The figure shows three views and two pictorial views of one solid part (mm, origin at its lowest corner). Answer the questions. A direction names the side the tool comes from. Coordinates: 2 decimals unless noted, no trailing zeros. Loops run counter-clockwise (first coordinate to the right, second up) from the corner with the lowest first, then second, coordinate; pieces in that order, holes last. Notation, with made-up numbers: (-3.5, 62) - (26.5, 62) arc R22 cw to (26.5, 101) - close; hole circle Ø2 at (28, 42). An arc over 180 degrees is marked (long way). Return JSON: item names as keys, results as strings. Group by question number.
1. Section A-A (z = 18) is taken. Write down the section's boundary in (x, y).
2. Each of these flat-tipped pins is pushed along its axis until it touches: P1, Ø2, axis at x = 8, z = 22, coming from the +Y side; P2, Ø10, axis at x = 27, y = 10, coming from the +Z side; P3, Ø4, axis at x = 27.5, y = 18, coming from the +Z side. Where does it stop, or does it pass through?
3. The mould has two halves that part along Y. Classify the marked faces 1, 2, 3 and 4: pulls with the +Y half, pulls with the -Y half, needs draft (parallel to the pull), parting line crosses it, or undercut.
4. Section C-C (x = 16) is taken. Write down the section's boundary in (y, z).
5. Section D-D (z = 3) is taken. Write down the section's boundary in (x, y).
6. Find the intervals of material crossed by line 1 along Y through (x, z) = (15, 3); line 2 along X through (y, z) = (7.5, 31); line 3 along X through (y, z) = (3, 19.5), in increasing order.
7. Which of the six approach directions +Z, -Z, +X, -X, +Y, -Y give full straight-line access (tool end or side, diameter ignored) to the marked faces 5, 6 and 7?
8. Section B-B (y = 17.5) is taken. Write down the section's boundary in (x, z).
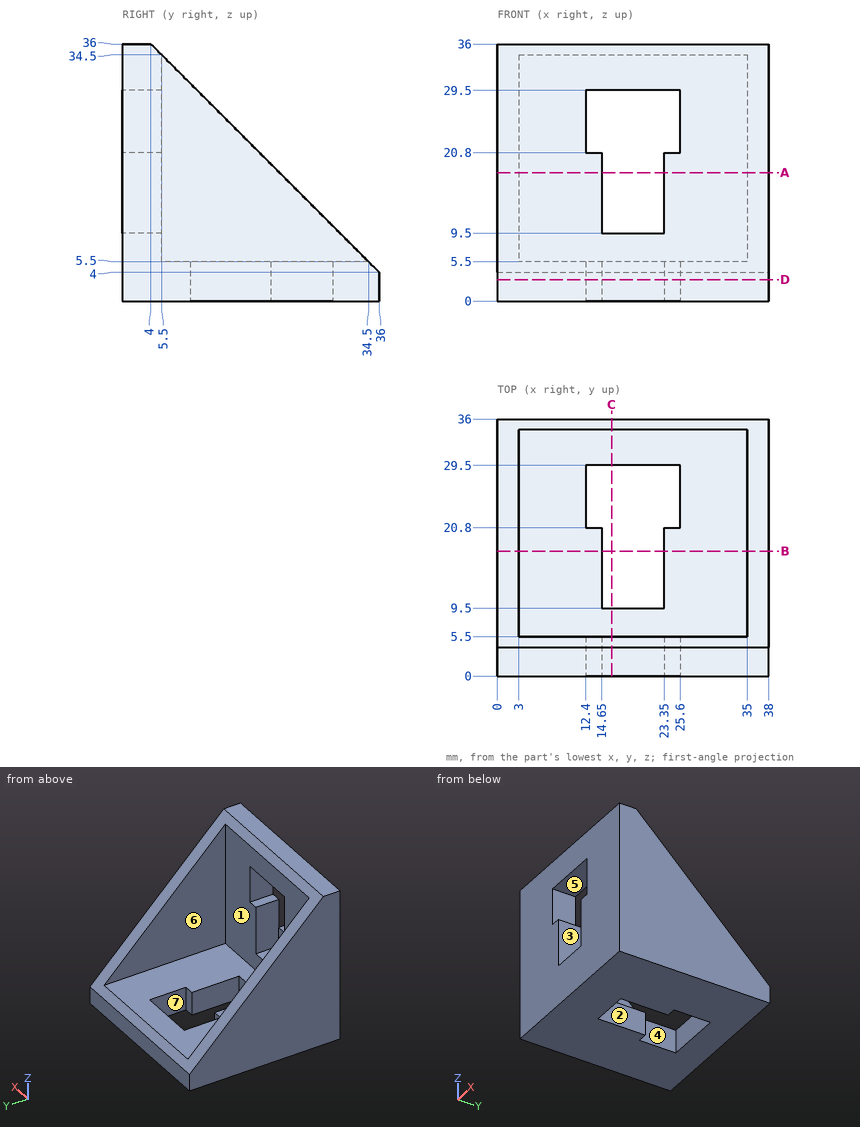
The answers:
{
 "1": {"outline": "(0, 0) - (14.65, 0) - (14.65, 5.5) - (3, 5.5) - (3, 22) - (0, 22) - close; (23.35, 0) - (38, 0) - (38, 22) - (35, 22) - (35, 5.5) - (23.35, 5.5) - close"},
 "2": {"P1": "stops at y = 5.5", "P2": "stops at z = 35", "P3": "stops at z = 5.5"},
 "3": {"face 1": "pulls with the +Y half", "face 2": "undercut", "face 3": "needs draft", "face 4": "undercut"},
 "4": {"outline": "(0, 0) - (9.5, 0) - (9.5, 5.5) - (5.5, 5.5) - (5.5, 9.5) - (0, 9.5) - close; (0, 29.5) - (5.5, 29.5) - (5.5, 34.5) - (4, 36) - (0, 36) - close; (29.5, 0) - (36, 0) - (36, 4) - (34.5, 5.5) - (29.5, 5.5) - close"},
 "5": {"outline": "(0, 0) - (38, 0) - (38, 36) - (0, 36) - close; hole (12.4, 20.8) - (14.65, 20.8) - (14.65, 9.5) - (23.35, 9.5) - (23.35, 20.8) - (25.6, 20.8) - (25.6, 29.5) - (12.4, 29.5) - close"},
 "6": {"line 1": "y = 0 to 9.5, 29.5 to 36", "line 2": "x = 0 to 3, 35 to 38", "line 3": "x = 0 to 14.65, 23.35 to 38"},
 "7": {"face 5": "+Y, -Y", "face 6": "+Z, +Y", "face 7": "+Z, -Z"},
 "8": {"outline": "(0, 0) - (14.65, 0) - (14.65, 5.5) - (3, 5.5) - (3, 22.5) - (0, 22.5) - close; (23.35, 0) - (38, 0) - (38, 22.5) - (35, 22.5) - (35, 5.5) - (23.35, 5.5) - close"}
}
